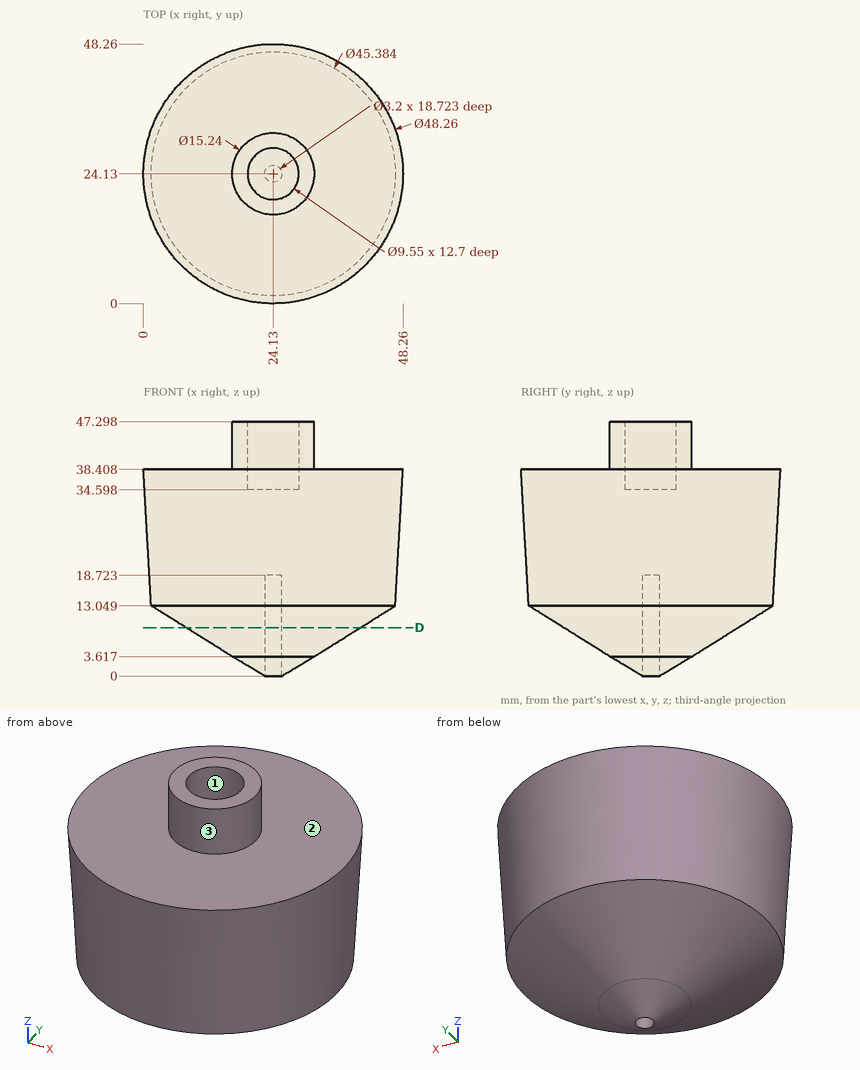
Verification items for this drawing (mm, ordinates from the low corner). Coordinates: 2 decimals unless noted, no trailing zeros. Loops run counter-clockwise (first coordinate to the right, second up) from the corner with the lowest first, then second, coordinate; pieces in that order, holes last.
Item 1: Thickness scan on line 1 (X direction, y = 24, z = 43); line 2 (Y direction, x = 24.13, z = 7.25) (1 decimal); line 3 (Y direction, x = 24.13, z = 7.75) (1 decimal). Record the ranges inside material, lowest first.
Item 2: Sectioned sample at D-D, the plane z = 9. Record the boundary of the cut face in (x, y), then the cut area to 3 significant figures.
Item 3: Release check for a two-part mould opening along Y. For the marked faces 1, 2 and 3 record: released by +Y, released by -Y, zero draft, split by the parting line, or undercut.
Item 4: Go/stop test with flat-tipped pins: pin 1 Ø6 at (x, y) = (13, 41) entering from -Z; pin 2 Ø5.5 at (x, y) = (24.13, 24.13) entering from +Z; pin 3 Ø2 at (x, z) = (9, 24.5) entering from -Y. Record where each tip stops, or that it passes through.
Check result:
1. line 1: x = 16.51 to 19.36, 28.9 to 31.75
1. line 2: y = 10.7 to 22.5, 25.7 to 37.6
1. line 3: y = 9.9 to 22.5, 25.7 to 38.4
2. outline: circle Ø32.44 at (24.13, 24.13); hole circle Ø3.2 at (24.13, 24.13)
2. area: 819 mm2
3. face 1: undercut
3. face 2: zero draft
3. face 3: split by the parting line
4. pin 1: stops at z = 9.62
4. pin 2: stops at z = 34.6
4. pin 3: stops at y = 5.55
